```python
from build123d import *

# Parameters (mm, degrees)
SKETCH1_R           = 7
BOSS_EXTRUDE1_DEPTH = 22
CUT_EXTRUDE1_START  = 14
CUT_EXTRUDE1_DEPTH  = 24
CUT_EXTRUDE2_START  = -19
SKETCH5_R           = 7
CUT_EXTRUDE2_DEPTH  = 19
SKETCH6_R           = 5.5
CUT_EXTRUDE3_DEPTH  = 91.60353194
CUT_EXTRUDE4_DEPTH  = 7
CUT_EXTRUDE5_DEPTH  = 25


with BuildPart() as part:
    # Sketch1 → Boss-Extrude1 (new, symmetric)
    with BuildSketch(Plane.XY):
        with BuildLine():
            Line((-14, 11), (-14, -7))
            Line((-14, -7), (-7, -14))
            Line((-7, -14), (25.575538911, -14))
            ThreePointArc((25.575538911, -14), (28.840774692, -15.213413768), (30.521177653, -18.264705882))
            ThreePointArc((30.521177653, -18.264705882), (32.858007856, -26.115672061), (37.296980053, -33))
            Line((37.296980053, -33), (43, -33))
            Line((43, -33), (72, 1))
            Line((72, 1), (72, 20))
            Line((72, 20), (67, 25))
            Line((67, 25), (43, 25))
            ThreePointArc((43, 25), (34.561098706, 15.982044142), (22.361380836, 14.057085233))
            Line((22.361380836, 14.057085233), (0, 18))
            Line((0, 18), (-7, 18))
            Line((-7, 18), (-14, 11))
        make_face()
        Circle(SKETCH1_R, mode=Mode.SUBTRACT)
    extrude(amount=BOSS_EXTRUDE1_DEPTH, both=True)

    # Sketch3 → Cut-Extrude1 (cut)
    with BuildSketch(Plane.XY.offset(CUT_EXTRUDE1_START)):
        with BuildLine():
            Line((72, 1), (72, 20))
            Line((72, 20), (67, 25))
            Line((67, 25), (43, 25))
            ThreePointArc((43, 25), (39.021244343, 19.259333621), (33.236936549, 15.344294617))
            ThreePointArc((33.236936549, 15.344294617), (44.184262982, -1.419294771), (61.764705882, -11))
            Line((61.764705882, -11), (72, 1))
        make_face()
    extrude(amount=-CUT_EXTRUDE1_DEPTH, mode=Mode.SUBTRACT)

    # Sketch5 → Cut-Extrude2 (cut)
    with BuildSketch(Plane.XY.offset(22).offset(CUT_EXTRUDE2_START)):
        Polygon((20, -14), (20, 14.473460386), (0, 18), (-7, 18), (-14, 11), (-14, -7), (-7, -14), align=None)
        Circle(SKETCH5_R, mode=Mode.SUBTRACT)
    extrude(amount=CUT_EXTRUDE2_DEPTH, mode=Mode.SUBTRACT)

    # Sketch6 → Cut-Extrude3 (cut, through all)
    with BuildSketch(Plane.XY.offset(22)):
        with Locations((58, 11)):
            Circle(SKETCH6_R)
    extrude(amount=-CUT_EXTRUDE3_DEPTH, mode=Mode.SUBTRACT)

    # Sketch7 → Cut-Extrude4 (cut)
    with BuildSketch(Plane.XY.offset(22)):
        with BuildLine():
            Line((22.187732658, 13.07227748), (21, 13.281706793))
            Line((21, 13.281706793), (21, -13))
            Line((21, -13), (25.575538911, -13))
            ThreePointArc((25.575538911, -13), (29.493821849, -14.456096521), (31.510305401, -18.117647059))
            ThreePointArc((31.510305401, -18.117647059), (33.672704892, -25.491599052), (37.758271763, -32))
            Line((37.758271763, -32), (42.538593943, -32))
            Line((42.538593943, -32), (71, 1.368545033))
            Line((71, 1.368545033), (71, 19.585786438))
            Line((71, 19.585786438), (66.585786438, 24))
            Line((66.585786438, 24), (43.636084685, 24))
            ThreePointArc((43.636084685, 24), (34.740005768, 14.948047079), (22.187732658, 13.07227748))
        make_face()
    extrude(amount=-CUT_EXTRUDE4_DEPTH, mode=Mode.SUBTRACT)

    # Sketch8 → Cut-Extrude5 (cut)
    with BuildSketch(Plane.XY.offset(15)):
        with BuildLine():
            Line((42.538593943, -32), (59.986847747, -11.543426575))
            ThreePointArc((59.986847747, -11.543426575), (43.310181683, -1.972127362), (32.646682943, 14.028208705))
            ThreePointArc((32.646682943, 14.028208705), (27.481076416, 12.851449437), (22.187732658, 13.07227748))
            Line((22.187732658, 13.07227748), (21, 13.281706793))
            Line((21, 13.281706793), (21, -13))
            Line((21, -13), (25.575538911, -13))
            ThreePointArc((25.575538911, -13), (29.493821849, -14.456096521), (31.510305401, -18.117647059))
            ThreePointArc((31.510305401, -18.117647059), (33.672704892, -25.491599052), (37.758271763, -32))
            Line((37.758271763, -32), (42.538593943, -32))
        make_face()
    extrude(amount=-CUT_EXTRUDE5_DEPTH, mode=Mode.SUBTRACT)


solid = part.part
```
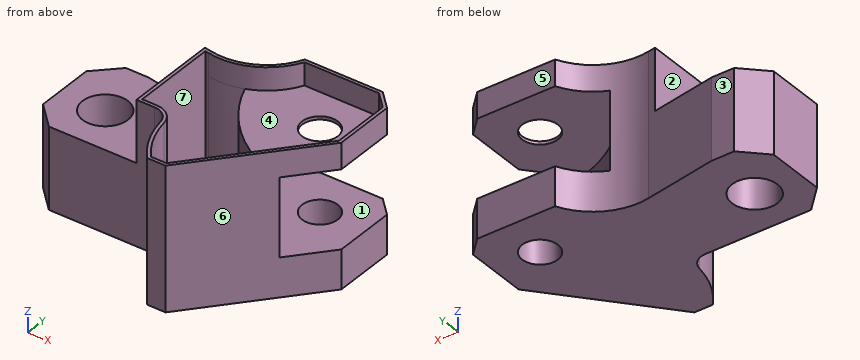
Work out the finished part from the listing and answer in its coordinate system (mm). Face numbers are marked on the shaded views. A direction names the side the tool comes from. Round coordinates to 2 decimals unless told otherwise and drop trailing zeros. Write each loop counter-clockwise with the first axis right and the second up, starting at its lowest first coordinate (ties: lowest second). Pieces come first, ordered by that corner, then holes.
1) A cutting plane is placed at D-D on x = -1. Determine the outline of the cut face in (y, z), and give its area (3 significant figures).
2) A cutting plane is placed at B-B on z = 10. Determine the outline of the cut face in (x, y).
3) Determine the mould class of the marked faces 5, 6 and 7 for opening direction Y: pulls with the +Y half, pulls with the -Y half, needs draft (parallel to the pull), parting line crosses it, or undercut.
4) A cutting plane is placed at A-A on z = -15. Determine the outline of the cut face in (x, y).
5) Which of the six approach directions +Z, -Z, +X, -X, +Y, -Y give full straight-line access (tool end or side, diameter ignored) to the marked faces 1, 2, 3 and 4?
6) A cutting plane is placed at C-C on y = 9. Determine the outline of the cut face in (x, z).
7) Consider probe 1 along Z at (x, y) = (41, 12.5); probe 2 along Z at (x, y) = (-7.5, 15); probe 3 along Y at (x, z) = (0, -17). Determine where each line is inside the solid, lowest interval first.
8) Flat-ended cylindrical pins translate along their axes: P1, Ø5, axis at x = 53.5, y = 16, coming from the +Z side; P2, Ø2, axis at x = 60, z = 7.5, coming from the -Y side; P3, Ø5, axis at x = 22.5, z = 10, coming from the +Y side; P4, Ø10, axis at x = 9.5, z = 10.5, coming from the -Y side. Find the tip coordinate at first contact, or state that the pin passes through.
Entries:
1. outline: (-14, -22) - (-6.93, -22) - (-6.93, 3) - (-14, 3) - close; (6.93, -22) - (18, -22) - (18, 3) - (6.93, 3) - close
1. area: 454 mm2
2. outline: (20, -14) - (25.58, -14) arc R5 cw to (30.52, -18.26) arc R29 ccw to (37.3, -33) - (43, -33) - (61.76, -11) arc R41 cw to (33.24, 15.34) arc R19 cw to (22.36, 14.06) - (20, 14.47) - close; hole (21, -13) - (25.58, -13) arc R6 cw to (31.51, -18.12) arc R28 ccw to (37.76, -32) - (42.54, -32) - (59.99, -11.54) arc R42 cw to (32.65, 14.03) arc R20 cw to (22.19, 13.07) - (21, 13.28) - close
3. face 5: pulls with the +Y half
3. face 6: pulls with the -Y half
3. face 7: undercut
4. outline: (-14, -7) - (-7, -14) - (25.58, -14) arc R5 cw to (30.52, -18.26) arc R29 ccw to (37.3, -33) - (43, -33) - (72, 1) - (72, 20) - (67, 25) - (43, 25) arc R19 cw to (22.36, 14.06) - (0, 18) - (-7, 18) - (-14, 11) - close; hole circle Ø14 at (0, 0); hole circle Ø11 at (58, 11)
5. face 1: +X, +Y
5. face 2: +Z, -X, +Y, -Y
5. face 3: +Z, -Z, -X, +Y
5. face 4: +Z
6. outline: (-14, -22) - (52.88, -22) - (52.88, -10) - (36.04, -10) - (36.04, 14) - (52.88, 14) - (52.88, 15) - (34.91, 15) - (34.91, -10) - (21, -10) - (21, 22) - (20, 22) - (20, 3) - (-14, 3) - close; (63.12, -22) - (72, -22) - (72, -10) - (63.12, -10) - close; (63.12, 14) - (72, 14) - (72, 22) - (71, 22) - (71, 15) - (63.12, 15) - close
7. probe 1: z = -22 to -10, 14 to 15
7. probe 2: z = -22 to 3
7. probe 3: y = -14 to -7, 7 to 18
8. P1: stops at z = 15
8. P2: stops at y = -14.24
8. P3: stops at y = 14.47
8. P4: passes through
